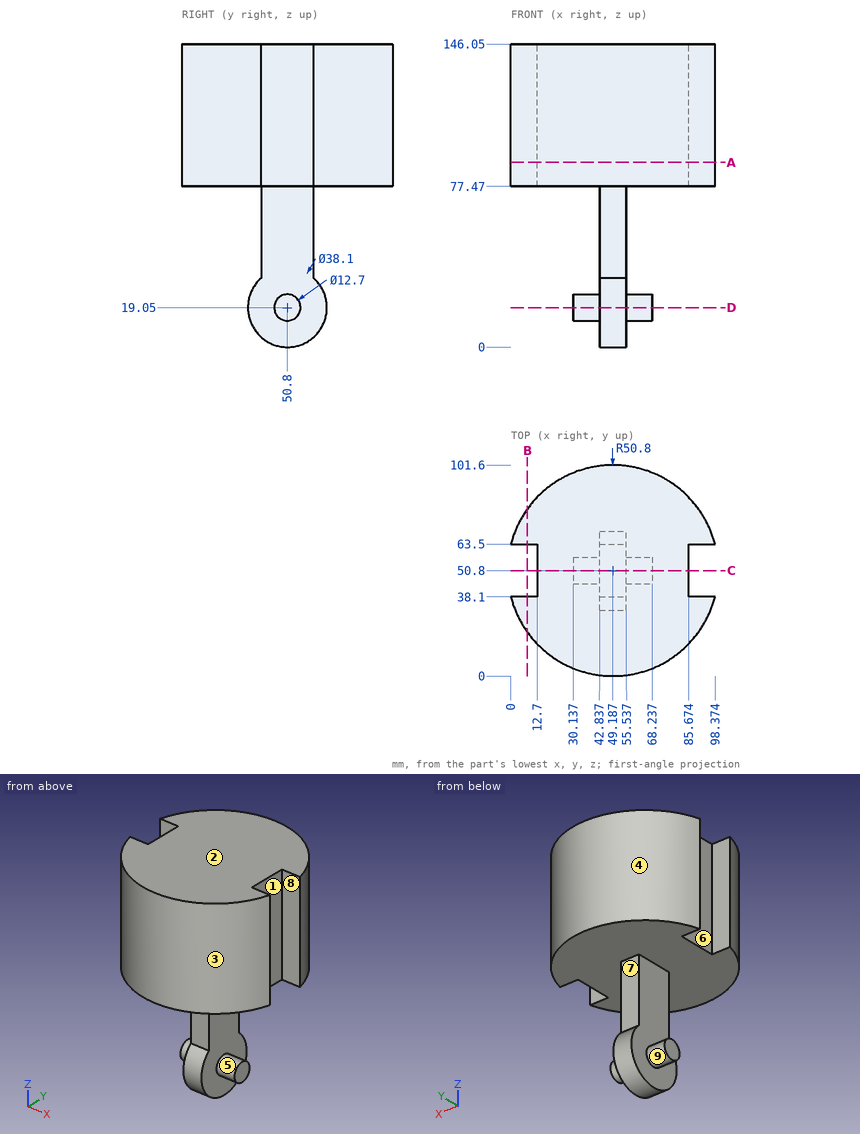
Check sheet for the drawn part. Datum: minimum x, y, z corner. Units: mm. A direction names the side the tool comes from. Give positions to 0.01 mm unless a question says otherwise; leave off trailing zeros. Write each loop counter-clockwise with the first axis right and the second up, starting at its lowest first coordinate (ties: lowest second). Pieces come first, ordered by that corner, then holes. Notation, with made-up numbers: (-8.75, -36.5) -> (17.25, -36.5) arc R36 ccw to (17.25, 1.5) -> close; hole circle Ø6 at (70, 24). An arc over 180 degrees is marked (long way). Use one line per item in the form item = value. Start each with the question number.
1. Section check B-B (x = 8). Record the cut outline in (y, z).
2. Access from +Z, -Z, +X, -X, +Y, -Y to the whole of each face (thin tool, end or side, straight path). Record for the marked faces 5, 6, 7, 8 and 9.
3. Thickness scan on line 1 along Z through (x, y) = (23, 80.5); line 2 along Y through (x, z) = (47.5, 135.5); line 3 along X through (y, z) = (58.5, 136). Record the ranges inside material, lowest first. Write a range as from..to.
4. Mould release check, pull along Y, two halves, no side actions. Record for the marked faces 1, 2, 3 and 4: pulls with the +Y half, pulls with the -Y half, needs draft (parallel to the pull), parting line crosses it, or undercut.
5. Section check C-C (y = 50.8). Record the cut outline in (x, z), and give its area (3 significant figures).
6. Go/stop test with flat-tipped pins: P1, Ø7.5, axis at y = 51.5, z = 126.5, coming from the -X side; P2, Ø6.5, axis at x = 48, z = 52, coming from the +Y side; P3, Ø6.5, axis at x = 94, z = 98, coming from the +Y side. Record where each tip stops, or that it passes through.
7. Section check D-D (z = 19.05). Record the cut outline in (x, y).
8. Section check A-A (z = 89). Record the cut outline in (x, y), and give its area (3 significant figures).
Conclusion:
q1.outline = (21.06, 77.47) -> (38.1, 77.47) -> (38.1, 146.05) -> (21.06, 146.05) -> close; (63.5, 77.47) -> (80.54, 77.47) -> (80.54, 146.05) -> (63.5, 146.05) -> close
q2.face_5 = +X
q2.face_6 = +Z, -Z, -X
q2.face_7 = +X, -X, +Y
q2.face_8 = +Z, -Z, +X
q2.face_9 = -X
q3.line_1 = 77.47..146.05
q3.line_2 = 0.03..101.57
q3.line_3 = 12.7..85.67
q4.face_1 = undercut
q4.face_2 = needs draft
q4.face_3 = pulls with the -Y half
q4.face_4 = pulls with the +Y half
q5.outline = (12.7, 77.47) -> (42.84, 77.47) -> (42.84, 25.4) -> (30.14, 25.4) -> (30.14, 12.7) -> (42.84, 12.7) -> (42.84, 0) -> (55.54, 0) -> (55.54, 12.7) -> (68.24, 12.7) -> (68.24, 25.4) -> (55.54, 25.4) -> (55.54, 77.47) -> (85.67, 77.47) -> (85.67, 146.05) -> (12.7, 146.05) -> close
q5.area = 6,310 mm²
q6.P1 = 12.7
q6.P2 = 63.5
q6.P3 = 80.01
q7.outline = (30.14, 44.45) -> (42.84, 44.45) -> (42.84, 31.75) -> (55.54, 31.75) -> (55.54, 44.45) -> (68.24, 44.45) -> (68.24, 57.15) -> (55.54, 57.15) -> (55.54, 69.85) -> (42.84, 69.85) -> (42.84, 57.15) -> (30.14, 57.15) -> close
q8.outline = (0, 38.1) arc R50.8 ccw to (98.37, 38.1) -> (85.67, 38.1) -> (85.67, 63.5) -> (98.37, 63.5) arc R50.8 ccw to (0, 63.5) -> (12.7, 63.5) -> (12.7, 38.1) -> close
q8.area = 7,410 mm²
